Work out the finished part from the listing and answer in its coordinate system (mm). Face numbers are marked on the shaded views. A direction names the side the tool comes from. Coordinates: 2 decimals unless noted, no trailing zeros. Order: outer loops, then holes, each group sorted by start corner. A loop starts at its lowest first (then second) coordinate and runs counter-clockwise, first axis right, second up.
1. A flat-ended cylindrical pin translates along its axis: pin 1 Ø1.5 at (y, z) = (43.5, -11.5) entering from -X. Find the tip coordinate at first contact, or state that the pin passes through.
2. Find the intervals of material crossed by probe 1 along Y at (x, z) = (5.25, -14); probe 2 along Z at (x, y) = (4, 7.5); probe 3 along Z at (x, y) = (2.25, 14), in increasing order.
3. The part is cut by section B-B, the plane y = 50. Give the vertices of the cut face in (x, z), then the cut area to 3 significant figures.
4. The part is cut by section C-C, the plane z = -3.5. Give the vertices of the cut face in (x, y).
5. A tool of negligible diameter and unlimited length cuts with its end or side. For the marked faces 1 and 2, from which of +Z, -Z, +X, -X, +Y, -Y can it reach the whole face along a straight path? Write none if from no direction.
6. The part is cut by section D-D, the plane x = 2.75. Give the vertices of the cut face in (y, z), then the cut area to 3 significant figures.
7. The part is cut by section A-A, the plane x = 5.75. Give the vertices of the cut face in (y, z), then the cut area to 3 significant figures.
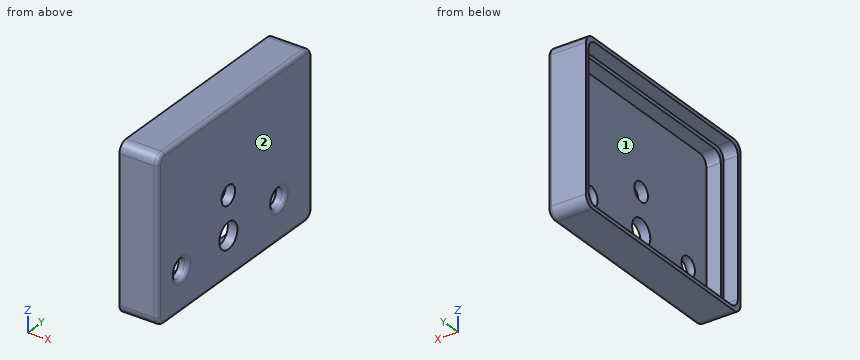
```python
from build123d import *

# Parameters (mm, degrees)
SKETCH1_W           = 43.18
SKETCH1_H           = 58.42
BOSS_EXTRUDE1_DEPTH = 10.16
SKETCH2_R           = 2.54
SKETCH2_R_2         = 3.429
CUT_EXTRUDE2_DEPTH  = 11.16
SKETCH3_W           = 39.116
SKETCH3_H           = 54.356
CUT_EXTRUDE3_DEPTH  = 7.62
SKETCH4_W           = 41.148
SKETCH4_H           = 56.388
CUT_EXTRUDE4_DEPTH  = 3.81
FILLET1_R           = 2.54
FILLET2_R           = 2.54
FILLET3_R           = 2.54
FILLET4_R           = 2.54
FILLET5_R           = 2.54
FILLET6_R           = 1
FILLET7_R           = 1
FILLET8_R           = 1


with BuildPart() as part:
    # Sketch1 → Boss-Extrude1 (new body)
    with BuildSketch(Plane(origin=(0, 0, 0), x_dir=(0, 0, -1), z_dir=(1, 0, 0))):
        with Locations((6.948060942, 29.21)):
            Rectangle(SKETCH1_W, SKETCH1_H)
    extrude(amount=BOSS_EXTRUDE1_DEPTH)

    # Sketch2 → Cut-Extrude2 (cut, through all)
    with BuildSketch(Plane.ZY):
        with Locations((-17.96692562, 8.890014802)):
            Circle(SKETCH2_R)
        with Locations((-17.881082197, 45.719807571)):
            Circle(SKETCH2_R)
        with Locations((-17.881082197, 26.669807571)):
            Circle(SKETCH2_R_2)
        with Locations((-7.710060942, 26.669807571)):
            Circle(SKETCH2_R)
    extrude(amount=-CUT_EXTRUDE2_DEPTH, mode=Mode.SUBTRACT)

    # Sketch3 → Cut-Extrude3 (cut)
    with BuildSketch(Plane.ZY):
        with Locations((-6.948060942, 29.21)):
            Rectangle(SKETCH3_W, SKETCH3_H)
    extrude(amount=-CUT_EXTRUDE3_DEPTH, mode=Mode.SUBTRACT)

    # Sketch4 → Cut-Extrude4 (cut)
    with BuildSketch(Plane.ZY):
        with Locations((-6.948060942, 29.21)):
            Rectangle(SKETCH4_W, SKETCH4_H)
    extrude(amount=-CUT_EXTRUDE4_DEPTH, mode=Mode.SUBTRACT)

    # Fillet1
    fillet1_edges = [part.edges().sort_by_distance(p)[0] for p in [
        (5.715, 2.032, -26.506060942),
        (1.905, 1.016, -27.522060942),
    ]]
    fillet(fillet1_edges, radius=FILLET1_R)

    # Fillet2
    fillet2_edges = [part.edges().sort_by_distance(p)[0] for p in [
        (5.715, 2.032, 12.609939058),
        (1.905, 1.016, 13.625939058),
    ]]
    fillet(fillet2_edges, radius=FILLET2_R)

    # Fillet3
    fillet3_edges = [part.edges().sort_by_distance(p)[0] for p in [
        (5.715, 56.388, 12.609939058),
        (1.905, 57.404, 13.625939058),
    ]]
    fillet(fillet3_edges, radius=FILLET3_R)

    # Fillet4
    fillet4_edges = [part.edges().sort_by_distance(p)[0] for p in [
        (5.715, 56.388, -26.506060942),
        (1.905, 57.404, -27.522060942),
    ]]
    fillet(fillet4_edges, radius=FILLET4_R)

    # Fillet5
    fillet5_edges = [part.edges().sort_by_distance(p)[0] for p in [
        (5.08, 58.42, 14.641939058),
        (5.08, 58.42, -28.538060942),
        (5.08, 0, -28.538060942),
        (5.08, 0, 14.641939058),
    ]]
    fillet(fillet5_edges, radius=FILLET5_R)

    # Fillet6
    fillet6_edges = [part.edges().sort_by_distance(p)[0] for p in [
        (10.16, 29.21, -28.538060942),
        (10.16, 0, -6.948060942),
        (10.16, 29.21, 14.641939058),
        (10.16, 58.42, -6.948060942),
        (10.16, 57.676051224, 13.897990282),
        (10.16, 57.676051224, -27.794112166),
        (10.16, 0.743948776, 13.897990282),
        (10.16, 0.743948776, -27.794112166),
    ]]
    fillet(fillet6_edges, radius=FILLET6_R)

    # Fillet7
    fillet7_edges = [part.edges().sort_by_distance(p)[0] for p in [
        (10.16, 45.719807571, -20.421082197),
    ]]
    fillet(fillet7_edges, radius=FILLET7_R)

    # Fillet8
    fillet8_edges = [part.edges().sort_by_distance(p)[0] for p in [
        (10.16, 8.890014802, -20.50692562),
    ]]
    fillet(fillet8_edges, radius=FILLET8_R)


solid = part.part
```
Geometry says:
1. pin 1: stops at x = 7.62
2. probe 1: y = 0 to 2.03, 56.39 to 58.42
2. probe 2: z = -28.54 to -26.51, 12.61 to 14.64
2. probe 3: z = -28.54 to -27.52, 13.63 to 14.64
3. outline: (0, -28.54) - (9.16, -28.54) arc R1 ccw to (10.16, -27.54) - (10.16, 13.64) arc R1 ccw to (9.16, 14.64) - (0, 14.64) - (0, 13.63) - (3.81, 13.63) - (3.81, 12.61) - (7.62, 12.61) - (7.62, -26.51) - (3.81, -26.51) - (3.81, -27.52) - (0, -27.52) - close
3. area: 132 mm2
4. outline: (0, 0) - (9.16, 0) arc R1 ccw to (10.16, 1) - (10.16, 57.42) arc R1 ccw to (9.16, 58.42) - (0, 58.42) - (0, 57.4) - (3.81, 57.4) - (3.81, 56.39) - (7.62, 56.39) - (7.62, 2.03) - (3.81, 2.03) - (3.81, 1.02) - (0, 1.02) - close
5. face 1: -X
5. face 2: +Z, -Z, +X, +Y, -Y
6. outline: (0, -26) arc R2.54 ccw to (2.54, -28.54) - (55.88, -28.54) arc R2.54 ccw to (58.42, -26) - (58.42, 12.1) arc R2.54 ccw to (55.88, 14.64) - (2.54, 14.64) arc R2.54 ccw to (0, 12.1) - close; hole (1.02, -24.98) arc R2.54 ccw to (3.56, -27.52) - (54.86, -27.52) arc R2.54 ccw to (57.4, -24.98) - (57.4, 11.09) arc R2.54 ccw to (54.86, 13.63) - (3.56, 13.63) arc R2.54 ccw to (1.02, 11.09) - close
6. area: 202 mm2
7. outline: (0, -26) arc R2.54 ccw to (2.54, -28.54) - (55.88, -28.54) arc R2.54 ccw to (58.42, -26) - (58.42, 12.1) arc R2.54 ccw to (55.88, 14.64) - (2.54, 14.64) arc R2.54 ccw to (0, 12.1) - close; hole (2.03, -23.97) arc R2.54 ccw to (4.57, -26.51) - (53.85, -26.51) arc R2.54 ccw to (56.39, -23.97) - (56.39, 10.07) arc R2.54 ccw to (53.85, 12.61) - (4.57, 12.61) arc R2.54 ccw to (2.03, 10.07) - close
7. area: 396 mm2
